Work out the finished part from the listing and answer in its coordinate system (mm). Face numbers are marked on the shaded views. A direction names the side the tool comes from. Coordinates: 2 decimals unless noted, no trailing zeros. Order: outer loops, then holes, each group sorted by start corner. A loop starts at its lowest first (then second) coordinate and runs counter-clockwise, first axis right, second up. Notation, with made-up numbers: (25, -10.75) - (63, -10.75) arc R35 cw to (63, 23.25) - close; hole circle Ø4 at (16, -23.75). An arc over 180 degrees is marked (long way). Answer as a JSON object with one key per item and string values. Group by question number.
1) The mould has two halves that part along X. Classify the marked faces 1, 2 and 3: released by +X, released by -X, zero draft, split by the parting line, or undercut.
2) Each of these flat-tipped pins is pushed along its axis until it touches: P1, Ø8, axis at x = 41.24, z = -23.81, coming from the +Y side; P2, Ø1, axis at y = 4.5, z = -12, coming from the -X side; P3, Ø2, axis at y = 6.5, z = 5, coming from the +X side. Where does it stop, or does it pass through?
3) A tool of negligible diameter and unlimited length cuts with its end or side. For the marked faces 4 and 5, from which of +Z, -Z, +X, -X, +Y, -Y can it reach the whole face along a straight path? Write none if from no direction.
4) Section A-A (z = 0) is taken. Give the vertices of the cut face in (x, y), plus the area to 3 significant figures.
5) Section B-B (x = 16.5) is taken. Give the vertices of the cut face in (y, z).
6) Section D-D (y = 5.75) is taken. Count the separate pieces of the cut face and the enclosed holes in it, plus the area to 3 significant figures.
7) Find the intervals of material crossed by line 1 along X through (y, z) = (9.5, 1); line 2 along Z through (x, y) = (-6, 12.25); line 3 along Z through (x, y) = (41, 7), in increasing order.
8) Section C-C (x = 0) is taken. Give the vertices of the cut face in (y, z) (3 decimals).
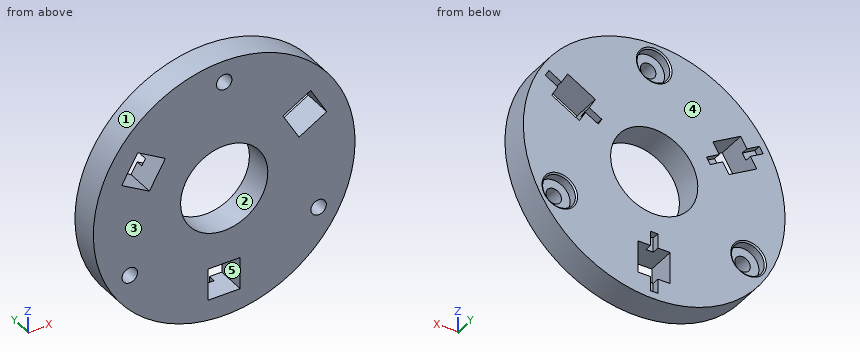
from build123d import *

# Parameters (mm, degrees)
SKETCH1_R                                    = 57.15
BOSS_EXTRUDE1_DEPTH                          = 12.7
SKETCH2_R                                    = 19.05
CUT_EXTRUDE1_DEPTH                           = 76.2
CBORE_FOR_1_4_BINDING_HEAD_MACHINE_S_2_COUNT = 2
CBORE_FOR_1_4_BINDING_HEAD_MACHINE_S_2_PITCH = 82.48891971
CBORE_FOR_1_4_BINDING_HEAD_MACHINE_S_3_COUNT = 2
CBORE_FOR_1_4_BINDING_HEAD_MACHINE_S_3_PITCH = 82.48891971
SKETCH5_W                                    = 13.97
SKETCH5_H                                    = 13.97
CUT_EXTRUDE2_DEPTH                           = 12.7
SKETCH7_W                                    = 3.175
SKETCH7_H                                    = 6.35
CUT_EXTRUDE4_DEPTH                           = 3.175


with BuildPart() as part:
    # Sketch1 → Boss-Extrude1 (new body)
    with BuildSketch(Plane(origin=(0, 0, 0), x_dir=(1, 0, 0), z_dir=(0, 1, 0))):
        with Locations(Location((0, 0, 0), (0, 0, 270))):
            Circle(SKETCH1_R)
    extrude(amount=BOSS_EXTRUDE1_DEPTH)

    # Sketch2 → Cut-Extrude1 (cut)
    with BuildSketch(Plane(origin=(0, 12.7, 0), x_dir=(1, 0, 0), z_dir=(0, 1, 0))):
        with Locations(Location((0, 0, 0), (0, 0, 270))):
            Circle(SKETCH2_R)
    extrude(amount=-CUT_EXTRUDE1_DEPTH, mode=Mode.SUBTRACT)

    # Sketch4 → CBORE for 1/4 Binding Head Machine Screw1 (revolve, cut)
    with BuildSketch(Plane(origin=(-41.244459855, 12.7, -23.8125), x_dir=(0, 0, 1), z_dir=(1, 0, 0))):
        Polygon((0, 0), (0, 12.7), (3.3782, 12.7), (3.3782, 4.191), (7.14375, 4.191), (7.14375, 0.532828266), (7.77875, 0), align=None)
    cbore_for_1_4_binding_head_machine_screw = revolve(axis=Axis((-41.244459855, 19.05, -23.8125), (0, -1, 0)), mode=Mode.SUBTRACT)

    # CBORE for 1_4 Binding Head Machine S 2: CBORE for 1/4 Binding Head Machine Screw1 ×2
    with Locations(*[(i * CBORE_FOR_1_4_BINDING_HEAD_MACHINE_S_2_PITCH, 0, 0) for i in range(1, CBORE_FOR_1_4_BINDING_HEAD_MACHINE_S_2_COUNT)]):
        add(cbore_for_1_4_binding_head_machine_screw, mode=Mode.SUBTRACT)

    # CBORE for 1_4 Binding Head Machine S 3: CBORE for 1/4 Binding Head Machine Screw1 ×2
    with Locations(*[Vector(0.4999999999999999, 0, 0.8660254037844388) * (i * CBORE_FOR_1_4_BINDING_HEAD_MACHINE_S_3_PITCH) for i in range(1, CBORE_FOR_1_4_BINDING_HEAD_MACHINE_S_3_COUNT)]):
        add(cbore_for_1_4_binding_head_machine_screw, mode=Mode.SUBTRACT)

    # Sketch5 → Cut-Extrude2 (cut)
    with BuildSketch(Plane(origin=(0, 12.7, 0), x_dir=(1, 0, 0), z_dir=(0, 1, 0))):
        Polygon((-44.771313472, -17.783146625), (-32.672938582, -10.798146625), (-25.687938582, -22.896521516), (-37.786313472, -29.881521516), align=None)
        Polygon((32.672938582, -10.798146625), (44.771313472, -17.783146625), (37.786313472, -29.881521516), (25.687938582, -22.896521516), align=None)
        with Locations((0, 40.67966814)):
            Rectangle(SKETCH5_W, SKETCH5_H)
    extrude(amount=-CUT_EXTRUDE2_DEPTH, mode=Mode.SUBTRACT)

    # Sketch7 → Cut-Extrude4 (cut)
    with BuildSketch(Plane(origin=(0, 12.7, 0), x_dir=(1, 0, 0), z_dir=(0, 1, 0))):
        with Locations((0, 50.83966814)):
            Rectangle(SKETCH7_W, SKETCH7_H)
        with Locations((0, 30.51966814)):
            Rectangle(SKETCH7_W, SKETCH7_H)
        Polygon((42.072563472, -22.457518742), (47.571824786, -25.632518742), (45.984324786, -28.382149399), (40.485063472, -25.207149399), align=None)
        Polygon((29.974188582, -15.472518742), (24.474927268, -12.297518742), (22.887427268, -15.047149399), (28.386688582, -18.222149399), align=None)
        Polygon((-40.485063472, -25.207149399), (-45.984324786, -28.382149399), (-47.571824786, -25.632518742), (-42.072563472, -22.457518742), align=None)
        Polygon((-28.386688582, -18.222149399), (-22.887427268, -15.047149399), (-24.474927268, -12.297518742), (-29.974188582, -15.472518742), align=None)
    extrude(amount=-CUT_EXTRUDE4_DEPTH, mode=Mode.SUBTRACT)


solid = part.part
Report:
{
 "1": {"face 1": "split by the parting line", "face 2": "undercut", "face 3": "zero draft"},
 "2": {"P1": "stops at y = 8.51", "P2": "stops at x = -55.98", "P3": "stops at x = 57.01"},
 "3": {"face 4": "+Z, -Z, +X, -X, +Y", "face 5": "+Y, -Y"},
 "4": {"outline": "(-57.15, 0) - (-19.05, 0) - (-19.05, 12.7) - (-57.15, 12.7) - close; (19.05, 0) - (57.15, 0) - (57.15, 12.7) - (19.05, 12.7) - close", "area": "968 mm²"},
 "5": {"outline": "(0, -54.72) - (12.7, -54.72) - (12.7, -9.52) - (0, -9.52) - close; (0, 9.52) - (12.7, 9.52) - (12.7, 54.72) - (0, 54.72) - close"},
 "6": {"separate pieces": "1", "enclosed holes": "7", "area": "8,430 mm²"},
 "7": {"line 1": "x = -57.14 to -19.02, 19.02 to 57.14", "line 2": "z = -56.83 to -47.66, -33.69 to -18.08, 18.08 to 43.57, 51.68 to 56.83", "line 3": "z = -39.81 to -27.18, -20.44 to 15.61, 24.32 to 39.81"},
 "8": {"outline": "(0, -57.15) - (12.7, -57.15) - (12.7, -54.015) - (9.525, -54.015) - (9.525, -47.665) - (0, -47.665) - close; (0, -33.695) - (9.525, -33.695) - (9.525, -27.345) - (12.7, -27.345) - (12.7, -19.05) - (0, -19.05) - close; (0, 19.05) - (12.7, 19.05) - (12.7, 39.846) - (12.167, 40.481) - (8.509, 40.481) - (8.509, 44.247) - (0, 44.247) - close; (0, 51.003) - (8.509, 51.003) - (8.509, 54.769) - (12.167, 54.769) - (12.7, 55.404) - (12.7, 57.15) - (0, 57.15) - close"}
}
